Read the model definition and answer for the solid it produces. Units are mm, in the model's axes. Face numbers are marked on the shaded views. A direction names the side the tool comes from. Coordinates: 2 decimals unless noted, no trailing zeros. Write each loop counter-clockwise with the first axis right and the second up, starting at its lowest first coordinate (ties: lowest second). Pieces come first, ordered by that corner, then holes. Notation, with made-up numbers: (35, -17) - (81, -17) arc R12 ccw to (81, -3) - close; hole circle Ø3 at (88, 32.5). An arc over 180 degrees is marked (long way). Use a Markdown table: item, result.
from build123d import *

# Parameters (mm, degrees)
SKETCH1_W                    = 101.6
SKETCH1_H                    = 50.8
BOSS_EXTRUDE1_DEPTH          = 4.7625
SKETCH3_W                    = 12.7
SKETCH3_H                    = 50.8
BOSS_EXTRUDE2_DEPTH          = 4.7625
F_10_0_1935_DIAMETER_HOLE1_D = 4.9149
SKETCH9_W                    = 6.35
SKETCH9_H                    = 3.175
CUT_EXTRUDE1_DEPTH           = 58.589283942


with BuildPart() as part:
    # Sketch1 → Boss-Extrude1 (new body)
    with BuildSketch(Plane(origin=(0, 0, 0), x_dir=(1, 0, 0), z_dir=(0, 1, 0))):
        Rectangle(SKETCH1_W, SKETCH1_H)
    extrude(amount=BOSS_EXTRUDE1_DEPTH)

    # Sketch3 → Boss-Extrude2 (add)
    with BuildSketch(Plane.XZ):
        with Locations((44.45, 0)):
            Rectangle(SKETCH3_W, SKETCH3_H)
    extrude(amount=BOSS_EXTRUDE2_DEPTH)

    # #10 (0.1935) Diameter Hole1 (through all)
    with Locations(Plane(origin=(0, 4.7625, 0), x_dir=(1, 0, 0), z_dir=(0, 1, 0))):
        with Locations((44.45, 7.139305), (44.45, -18.260695)):
            Hole(F_10_0_1935_DIAMETER_HOLE1_D / 2)

    # Sketch9 → Cut-Extrude1 (cut, through all)
    with BuildSketch(Plane(origin=(0, 4.7625, 0), x_dir=(1, 0, 0), z_dir=(0, 1, 0))):
        with Locations((24.731908969, 23.8125)):
            Rectangle(SKETCH9_W, SKETCH9_H)
        with Locations((-18.099171267, 23.8125)):
            Rectangle(SKETCH9_W, SKETCH9_H)
        with Locations((-23.921416816, -23.8125)):
            Rectangle(SKETCH9_W, SKETCH9_H)
        with Locations((14.878103248, -23.8125)):
            Rectangle(SKETCH9_W, SKETCH9_H)
    extrude(amount=-CUT_EXTRUDE1_DEPTH, mode=Mode.SUBTRACT)


solid = part.part
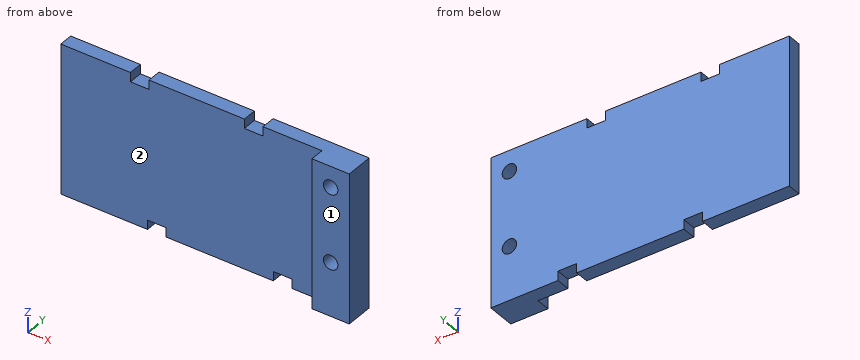
(1) For the marked faces 1 and 2, determine the directions among +Z, -Z, +X, -X, +Y, -Y from which every point of the face is accessible in a straight line to the end or side of a thin tool.
Report:
| item | result |
|---|---|
| face 1 | +Z, -Z, +X, -X, -Y |
| face 2 | +Z, -Z, -X, -Y |
(2) Straight lines are drawn through the part: L1, parallel to Z at x = 44.45, y = 1.5; L2, parallel to Y at x = -14, z = -9; L3, parallel to X at y = -2, z = -13. For each, find the intervals that lie inside material, in ascending order.
Report:
| item | result |
|---|---|
| L1 | z = -25.4 to -9.6, -4.68 to 15.8, 20.72 to 25.4 |
| L2 | y = 0 to 4.76 |
| L3 | x = 38.1 to 50.8 |
(3) A cutting plane is placed at B-B, the plane y = 2.5. Write down the section's boundary in (x, z) (3 decimals), and give its area (3 significant figures).
Report:
| item | result |
|---|---|
| outline | (-50.8, -25.4) - (-21.274, -25.4) - (-21.274, -22.225) - (-14.924, -22.225) - (-14.924, -25.4) - (21.557, -25.4) - (21.557, -22.225) - (27.907, -22.225) - (27.907, -25.4) - (50.8, -25.4) - (50.8, 25.4) - (18.053, 25.4) - (18.053, 22.225) - (11.703, 22.225) - (11.703, 25.4) - (-20.746, 25.4) - (-20.746, 22.225) - (-27.096, 22.225) - (-27.096, 25.4) - (-50.8, 25.4) - close; hole circle Ø4.915 at (44.45, -7.139); hole circle Ø4.915 at (44.45, 18.261) |
| area | 5,040 mm² |
(4) A cutting plane is placed at A-A, the plane x = 44.45. Write down the section's boundary in (y, z), and give its area (3 significant figures).
Report:
| item | result |
|---|---|
| outline | (-4.76, -25.4) - (4.76, -25.4) - (4.76, -9.6) - (-4.76, -9.6) - close; (-4.76, -4.68) - (4.76, -4.68) - (4.76, 15.8) - (-4.76, 15.8) - close; (-4.76, 20.72) - (4.76, 20.72) - (4.76, 25.4) - (-4.76, 25.4) - close |
| area | 390 mm² |
(5) Each of these flat-tipped pins is pushed along its axis until it touches: P1, Ø2.5, axis at x = 14.5, y = 2, coming from the +Z side (3 decimals); P2, Ø4, axis at x = -8, z = -2.5, coming from the -Y side; P3, Ø2.5, axis at x = -16.5, y = 3.5, coming from the -Z side (3 decimals). Where does it stop, or does it pass through?
Report:
| item | result |
|---|---|
| P1 | stops at z = 22.225 |
| P2 | stops at y = 0 |
| P3 | stops at z = -22.225 |
(6) A cutting plane is placed at D-D, the plane x = -29.5. Write down the section's boundary in (y, z), and give its area (3 significant figures).
Report:
| item | result |
|---|---|
| outline | (0, -25.4) - (4.76, -25.4) - (4.76, 25.4) - (0, 25.4) - close |
| area | 242 mm² |
(7) A cutting plane is placed at C-C, the plane z = 14.5. Write down the section's boundary in (x, y).
Report:
| item | result |
|---|---|
| outline | (-50.8, 0) - (38.1, 0) - (38.1, -4.76) - (50.8, -4.76) - (50.8, 4.76) - (-50.8, 4.76) - close |
